CAD build for the part. Positions are in the model's coordinates, mm. Face numbers are marked on the shaded views. Coordinates: 2 decimals unless noted, no trailing zeros. Order: outer loops, then holes, each group sorted by start corner. A loop starts at its lowest first (then second) coordinate and runs counter-clockwise, first axis right, second up. Notation, with made-up numbers: M 23.5,-15 L 56.5,-15 A17 ccw 56.5,-5 Z; hole C -4.75,69 d5. An arc over 180 degrees is marked long. One line per item, written item: value.
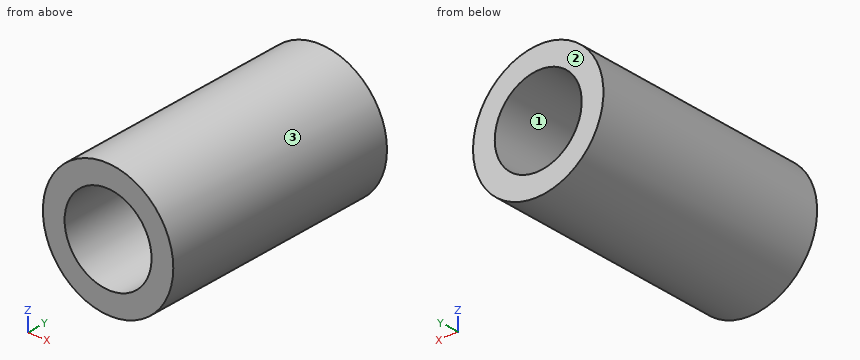
Autodesk Fusion 360 part; units mm, degrees
sketch "スケッチ1" plane through (0, 0, 0) normal (0, 1, 0) x (1, 0, 0)
  circle A0 centre (0, 0) radius 1.3
  circle A1 centre (0, 0) radius 2.5
  circle A2 centre (0, 0) radius 1.5
  dimension "d1" = 2.6
extrude "押し出し2" add sketch "スケッチ1" along normal blind 11 contours A1 makes body 1
extrude "押し出し1" add sketch "スケッチ1" along normal blind 11 separate body contours A1 | A2 makes body 2
sketch "スケッチ2" plane through (0, 0, 0) normal (0, 1, 0) x (1, 0, 0)
  circle A0 centre (0, 0) radius 2
  circle A1 centre (0, 0) radius 3
extrude "押し出し3" add sketch "スケッチ2" along normal blind 11 separate body makes body 3
hidden bodies 1 2
Q1. Slice it at B-B (x = 0). List the corners of the cut face in (y, z), plus the area to 3 significant figures.
Recorded:
outline: M 0,-3 L 11,-3 L 11,-2 L 0,-2 Z; M 0,2 L 11,2 L 11,3 L 0,3 Z
area: 22.0 mm^2
Q2. Slice it at A-A (z = 0). List the corners of the cut face in (x, y).
Recorded:
outline: M -3,0 L -2,0 L -2,11 L -3,11 Z; M 2,0 L 3,0 L 3,11 L 2,11 Z
Q3. Mould opens along Z. For the marked faces 1, 2 and 3 say: released by +Z, released by -Z, zero draft, split by the parting line, or undercut.
Recorded:
face 1: undercut
face 2: zero draft
face 3: split by the parting line
Q4. Pin check, flat tips, straight feed: pin 1 Ø1.5 at (x, z) = (-1.5, -1.5) entering from -Y; pin 2 Ø2 at (x, y) = (2, 5.5) entering from +Z. Stop position of each tip, or through.
Recorded:
pin 1: stops at y = 0
pin 2: stops at z = 2.83
Q5. Slice it at C-C (y = 9.75). List the corners of the cut face in (x, z), plus the area to 3 significant figures.
Recorded:
outline: C 0,0 d6; hole C 0,0 d4
area: 15.7 mm^2
Q6. Slice it at D-D (z = 2.15). List the corners of the cut face in (x, y), plus the area to 3 significant figures.
Recorded:
outline: M -2.09,0 L 2.09,0 L 2.09,11 L -2.09,11 Z
area: 46.0 mm^2
Q7. Drill centre lines: line 1 along Z through (x, y) = (0, 8.5); line 2 along X through (y, z) = (4.25, 1.8). Where is each one in solid material? Low to high.
Recorded:
line 1: z = -3 to -2, 2 to 3
line 2: x = -2.4 to -0.87, 0.87 to 2.4
